from build123d import *

# Parameters (mm, degrees)
F1_DEPTH = 25
F3_D     = 20
F3_DEPTH = 10
F3_TIP   = 6.0086061903
F4_R     = 5


with BuildPart() as f1:
    # F0 (on Front) → F1 (new body)
    with BuildSketch(Plane.XZ):
        with BuildLine():
            Line((-135.8573855514, 30), (-135.8573855514, 0))
            Line((-135.8573855514, 0), (140.1426144486, 0))
            Line((140.1426144486, 0), (140.1426144486, 30))
            ThreePointArc((140.1426144486, 30), (115.3358512852, 41.5398552549), (95.1426144486, 60))
            Line((95.1426144486, 60), (-90.8573855514, 60))
            ThreePointArc((-90.8573855514, 60), (-111.0506223879, 41.5398552549), (-135.8573855514, 30))
        make_face()
    extrude(amount=-F1_DEPTH)

    # F3
    with Locations(Plane(origin=(0, 0, 0), x_dir=(1, 0, 0), z_dir=(0, 0, -1))):
        with Locations((-66.8573855514, -12.5), (2.1426144486, -12.5), (71.1426144486, -12.5)):
            Hole(F3_D / 2, depth=F3_DEPTH)
            with Locations((0, 0, -(F3_DEPTH + F3_TIP / 2))):  # 118° drill point
                Cone(0, F3_D / 2, F3_TIP, mode=Mode.SUBTRACT)

    # F4
    f4_edges = [f1.edges().sort_by_distance(p)[0] for p in [
        (140.142614, 12.5, 0),
        (140.142614, 12.5, 30),
        (140.142614, 0, 15),
        (140.142614, 25, 15),
        (-135.857386, 12.5, 30),
        (-135.857386, 12.5, 0),
        (-135.857386, 0, 15),
        (-135.857386, 25, 15),
        (-90.857386, 12.5, 60),
        (-111.050622, 0, 41.539855),
        (-111.050622, 25, 41.539855),
        (95.142614, 12.5, 60),
        (2.142614, 0, 60),
        (2.142614, 25, 60),
        (115.335851, 0, 41.539855),
        (115.335851, 25, 41.539855),
    ]]
    fillet(f4_edges, radius=F4_R)


solid = f1.part
Model file for the job. Use its own axes, mm. A direction names the side the tool comes from. Give positions to 0.01 mm unless a question says otherwise; leave off trailing zeros. Return JSON: item names as keys, results as strings.
1) Pull direction X, two halves, no side cores. Call faces 3 (the cylindrical face through (-134.43, 23.5, 12.98)), 4 (the cylindrical face through (10.08, 18.58, 5.07)), 5 (the cylindrical face through (138.639, 12.675, 1.426)): pulls with the +X half, pulls with the -X half, needs draft (parallel to the pull), parting line crosses it, or undercut.
Geometry says:
{"face 3": "pulls with the -X half", "face 4": "undercut", "face 5": "pulls with the +X half"}
2) Probe line 1 (Z direction, x = 43, y = 20.5); line 2 (Z direction, x = 100, y = 2.75); line 3 (X direction, y = 7, z = 35). List the from-to ranges inside material, lowest first. Write a range as from..to.
Geometry says:
{"line 1": "0..59.97", "line 2": "0..53.67", "line 3": "-122.63..126.92"}
3) Flat gauge pins, fed straight in: P1, Ø12, axis at x = -66.86, y = 12.5, coming from the -Z side; P2, Ø2, axis at y = 21.5, z = 18, coming from the +X side; P3, Ø1.5, axis at y = 7, z = 44, coming from the -X side. Where does each tip first touch, or does it go through?
Geometry says:
{"P1": "z = 12.4", "P2": "x = 140.12", "P3": "x = -108.58"}
4) 3-axis set-ups, long thin cutter, end or side, ignore diameter. For faces 1 (the cylindrical face through (-134.43, 12.68, 1.5)), 2 (the cylindrical face through (-56.867, 12.06, 5.07)): which of +Z, -Z, +X, -X, +Y, -Y reach the whole face in a straight line?
Geometry says:
{"face 1": "-Z, -X, +Y, -Y", "face 2": "-Z"}
